Source: CAD feature listing. Evaluate the final solid. Frame: model axes, mm. A direction names the side the tool comes from. Coordinates: 2 decimals unless noted, no trailing zeros. Write each loop counter-clockwise with the first axis right and the second up, starting at its lowest first coordinate (ties: lowest second). Pieces come first, ordered by that corner, then holes. Notation, with made-up numbers: (-4, -25.5) - (37, -25.5) arc R14 ccw to (37, -1.5) - close; hole circle Ø8 at (47.5, 18). An arc over 180 degrees is marked (long way). One line per item, written item: value.
from build123d import *

# Parameters (mm, degrees)
BOSS_EXTRUDE1_DEPTH = 0.254
SKETCH3_W           = 3.81
SKETCH3_H           = 7.112
BOSS_EXTRUDE2_DEPTH = 1.016
BOSS_EXTRUDE3_DEPTH = 3.81
CUT_EXTRUDE1_DEPTH  = 3.81
CUT_EXTRUDE3_DEPTH  = 3.81
SKETCH9_W           = 5.334
SKETCH9_H           = 0.254
BOSS_EXTRUDE4_DEPTH = 2.032
BOSS_EXTRUDE5_DEPTH = 2.032
BOSS_EXTRUDE6_DEPTH = 7.62
SKETCH15_W          = 0.254
SKETCH15_H          = 13.969943058
CUT_EXTRUDE4_DEPTH  = 24.162808673
FILLET1_R           = 0.254
FILLET2_R           = 0.254
SKETCH16_R          = 2.159
CUT_EXTRUDE5_DEPTH  = 7.62
CUT_EXTRUDE6_DEPTH  = 7.62


with BuildPart() as part:
    # Sketch2 → Boss-Extrude1 (new body)
    with BuildSketch(Plane.XY):
        with BuildLine():
            Line((0, 7.62), (0, 0))
            Line((0, 0), (3.81, 0))
            Line((3.81, 0), (3.81, 13.716))
            Line((3.81, 13.716), (-0.967403026, 34.249561414))
            Line((-0.967403026, 34.249561414), (0.377089259, 44.819493706))
            Line((0.377089259, 44.819493706), (-2.162910741, 44.819493706))
            Line((-2.162910741, 44.819493706), (-2.162910741, 47.994493706))
            ThreePointArc((-2.162910741, 47.994493706), (-0.584766227, 50.738701708), (2.580823154, 50.754873928))
            Line((2.580823154, 50.754873928), (9.612257003, 59.112446663))
            Line((9.612257003, 59.112446663), (17.936769995, 72.485209152))
            Line((17.936769995, 72.485209152), (16.427333856, 73.424829575))
            ThreePointArc((16.427333856, 73.424829575), (15.208368205, 71.757285785), (13.146272514, 71.877039345))
            ThreePointArc((13.146272514, 71.877039345), (12.149333877, 73.408865168), (12.684466147, 75.156437899))
            Line((12.684466147, 75.156437899), (11.175030007, 76.096058323))
            Line((11.175030007, 76.096058323), (2.122651116, 61.554028899))
            Line((2.122651116, 61.554028899), (-3.456202303, 52.591981292))
            ThreePointArc((-3.456202303, 52.591981292), (-6.537615376, 44.154125487), (-6.264635755, 35.175372833))
            Line((-6.264635755, 35.175372833), (-4.777403026, 34.249561414))
            Line((-4.777403026, 34.249561414), (0, 13.716))
            Line((0, 13.716), (0, 7.62))
        make_face()
    extrude(amount=BOSS_EXTRUDE1_DEPTH)

    # Sketch3 → Boss-Extrude2 (add)
    with BuildSketch(Plane.XY.offset(0.254)):
        with Locations((1.905, 3.556)):
            Rectangle(SKETCH3_W, SKETCH3_H)
    extrude(amount=BOSS_EXTRUDE2_DEPTH)

    # Sketch4 → Boss-Extrude3 (add)
    with BuildSketch(Plane(origin=(3.81, 0, 0), x_dir=(0, 0, -1), z_dir=(1, 0, 0))):
        Polygon((-1.27, 7.112), (-0.254, 8.128), (-0.254, 7.112), align=None)
    extrude(amount=-BOSS_EXTRUDE3_DEPTH)

    # Sketch5 → Cut-Extrude1 (cut)
    with BuildSketch(Plane(origin=(3.81, 0, 0), x_dir=(0, 0, -1), z_dir=(1, 0, 0))):
        Polygon((0, 0), (-1.016, 0), (-1.016, 7.006789755), (0, 8.022789755), align=None)
    extrude(amount=-CUT_EXTRUDE1_DEPTH, mode=Mode.SUBTRACT)

    # Sketch7 → Cut-Extrude3 (cut)
    with BuildSketch(Plane.XY.offset(1.27)):
        Polygon((0, 0.508), (0.381, 0), (0.762, 0.508), (1.143, 0), (1.524, 0.508), (1.905, 0), (2.286, 0.508), (2.667, 0), (3.048, 0.508), (3.429, 0), (3.81, 0.508), (3.81, 0), (0, 0), align=None)
    extrude(amount=-CUT_EXTRUDE3_DEPTH, mode=Mode.SUBTRACT)

    # Sketch9 → Boss-Extrude4 (add)
    with BuildSketch(Plane.XY.offset(0.254)):
        with Locations((0.504089259, 44.692493706)):
            Rectangle(SKETCH9_W, SKETCH9_H)
    extrude(amount=-BOSS_EXTRUDE4_DEPTH)

    # Sketch10 → Boss-Extrude5 (add)
    with BuildSketch(Plane(origin=(0, 0, 0), x_dir=(-1, 0, 0), z_dir=(0, 0, -1))):
        with BuildLine():
            Line((5.928887496, 35.253489079), (6.264635755, 35.175372833))
            ThreePointArc((6.264635755, 35.175372833), (6.537615376, 44.154125487), (3.456202303, 52.591981292))
            Line((3.456202303, 52.591981292), (-3.926529596, 64.451836675))
            Line((-3.926529596, 64.451836675), (-4.148451246, 64.313690973))
            Line((-4.148451246, 64.313690973), (3.202180271, 52.505402665))
            ThreePointArc((3.202180271, 52.505402665), (6.248425743, 44.145431055), (5.928887496, 35.253489079))
        make_face()
    extrude(amount=BOSS_EXTRUDE5_DEPTH)

    # Sketch13 → Boss-Extrude6 (add)
    with BuildSketch(Plane(origin=(-19.592819025, 12.196483461, 0), x_dir=(0, 0, -1), z_dir=(0.84895171, -0.528470429, 0))):
        with BuildLine():
            Line((0, 56.791551712), (2.032, 56.791551712))
            ThreePointArc((2.032, 56.791551712), (2.930025612, 57.1635261), (3.302, 58.061551712))
            Line((3.302, 58.061551712), (3.302, 71.01549477))
            Line((3.302, 71.01549477), (3.048, 71.01549477))
            Line((3.048, 71.01549477), (3.048, 58.117392676))
            ThreePointArc((3.048, 58.117392676), (2.73406505, 57.359486662), (1.976159036, 57.045551712))
            Line((1.976159036, 57.045551712), (0, 57.045551712))
            Line((0, 57.045551712), (0, 56.791551712))
        make_face()
    extrude(amount=-BOSS_EXTRUDE6_DEPTH)

    # Sketch15 → Cut-Extrude4 (cut, through all)
    with BuildSketch(Plane(origin=(-19.592819025, 12.196483461, 0), x_dir=(0, 0, -1), z_dir=(0.84895171, -0.528470429, 0))):
        with Locations((-0.127, 64.030523241)):
            Rectangle(SKETCH15_W, SKETCH15_H)
    extrude(amount=-CUT_EXTRUDE4_DEPTH, mode=Mode.SUBTRACT)

    # Fillet1
    fillet1_edges = [part.edges().sort_by_distance(p)[0] for p in [
        (7.307414636, 62.646436259, 0.254),
    ]]
    fillet(fillet1_edges, radius=FILLET1_R)

    # Fillet2
    fillet2_edges = [part.edges().sort_by_distance(p)[0] for p in [
        (7.284143972, 62.361729674, 0),
    ]]
    fillet(fillet2_edges, radius=FILLET2_R)

    # Sketch16 → Cut-Extrude5 (cut)
    with BuildSketch(Plane.XY.offset(-3.048)):
        with Locations((14.737858035, 74.315544717)):
            Circle(SKETCH16_R)
    extrude(amount=-CUT_EXTRUDE5_DEPTH, mode=Mode.SUBTRACT)

    # Sketch17 → Cut-Extrude6 (cut)
    with BuildSketch(Plane.XY.offset(-3.048)):
        with BuildLine():
            Line((12.664355285, 67.379861092), (12.395892307, 66.948593623))
            ThreePointArc((12.395892307, 66.948593623), (9.946835744, 66.378777907), (9.377020028, 68.82783447))
            Line((9.377020028, 68.82783447), (9.645483006, 69.259101939))
            ThreePointArc((9.645483006, 69.259101939), (12.094539569, 69.828917655), (12.664355285, 67.379861092))
        make_face()
    extrude(amount=-CUT_EXTRUDE6_DEPTH, mode=Mode.SUBTRACT)


solid = part.part
1) Section query D-D on y = 5. Output: boundary loops of the cut face in (x, z).
Values found:
outline: (0, 1.02) - (3.81, 1.02) - (3.81, 1.27) - (0, 1.27) - close
2) Reachability of faces 5 (the flat face through (1, 44.819, -1)), 6 (the flat face through (-1, 41, 0.254)), 7 (the flat face through (7.365, 62.611, -1.002)) from +Z, -Z, +X, -X, +Y, -Y: full face, straight path, thin tool, end or side. Return the list, or none.
Values found:
face 5: +Z, -Z, +X
face 6: +Z, +X, -X, +Y
face 7: +Z, +X, +Y
3) Contact query for flat-ended pins moving along their axis: P1, Ø6, axis at x = 11, y = 55.5, coming from the +Z side; P2, Ø4, axis at x = 11.5, y = 71.5, coming from the +Z side; P3, Ø1, axis at x = 5, z = 0.5, coming from the +Y side; P4, Ø0.6, axis at x = 0.5, z = -1, coming from the +Y side. Output: stop coordinate, or through.
Values found:
P1: through
P2: z = -3.05
P3: y = 64.25
P4: y = 59.43
4) Draft query along Y for faces 1 (the flat face through (2, 4, 1.27)), 2 (the cylindrical face through (7.2, 62.33, -0.08)), 3 (the flat face through (0.525, 58.492, -1.002)), 4 (the cylindrical face through (-6.557, 44.029, -0.873)). Return one class per face: released by +Y, released by -Y, zero draft, split by the parting line, or undercut.
Values found:
face 1: zero draft
face 2: released by -Y
face 3: undercut
face 4: split by the parting line
5) Section query C-C on x = 13.75. Output: boundary loops of the cut face in (y, z), then the cut area to 3 significant figures.
Values found:
outline: (65.76, -3.3) - (72.4, -3.3) - (72.4, -3.05) - (65.76, -3.05) - close
area: 1.69 mm2
6) Section query A-A on y = 56. Output: boundary loops of the cut face in (x, z), then the cut area to 3 significant figures.
Values found:
outline: (-1.33, -2.03) - (-1.03, -2.03) - (-1.03, 0) - (6.99, 0) - (6.99, 0.25) - (-1.33, 0.25) - close
area: 2.74 mm2
7) Material intervals for line 1 (Y direction, x = -1.75, z = -1.15); line 2 (X direction, y = 45.5, z = 0.1); line 3 (Z direction, x = -2.25, y = 31.5), sorted ascending.
Values found:
line 1: 44.57 to 44.82, 54.84 to 55.33
line 2: -6.28 to -2.16
line 3: 0 to 0.25
8) Section query B-B on y = 47. Output: boundary loops of the cut face in (x, z), then the cut area to 3 significant figures.
Values found:
outline: (-5.9, -2.03) - (-5.61, -2.03) - (-5.61, 0) - (-2.16, 0) - (-2.16, 0.25) - (-5.9, 0.25) - close
area: 1.53 mm2
